Part model, mm, in its own coordinate system. Face numbers are marked on the shaded views. A direction names the side the tool comes from. Round coordinates to 2 decimals unless told otherwise and drop trailing zeros. Write each loop counter-clockwise with the first axis right and the second up, starting at its lowest first coordinate (ties: lowest second). Pieces come first, ordered by that corner, then holes. Notation, with made-up numbers: M -23.5,-21 L -2.5,-21 A18 cw -2.5,-9 Z; hole C 71.5,38 d7. An arc over 180 degrees is marked long. Answer as a JSON object with one key per item and string values. Group by question number.
1. Band-saw the part on D-D, the plane z = 9. Write the cut outline in (x, y) (3 decimals).
2. Which spindle directions (+Z, -Z, +X, -X, +Y, -Y) get a long thin tool onto all of the face, cutting with end or side? Do the marked faces 5 and 6. Say none if no direction does.
3. Two-plate mould, pull along Z, no slides. Class the marked faces 1, 2, 3 and 4: +Z half, -Z half, draft (parallel to the pull), parting line (faces both ways), or undercut.
4. Band-saw the part on C-C, the plane x = 3.25. Write the cut outline in (y, z).
5. Drill centre lines: line 1 (Z direction, x = 2.5, y = 1.25); line 2 (Y direction, x = 4.5, z = 9.25) (3 decimals); line 3 (X direction, y = 2.5, z = 1.25). Where is each one in solid material? Low to high. Write a range as from..to.
6. Band-saw the part on A-A, the plane x = 7.25. Write the cut outline in (y, z) (3 decimals).
7. Drop flat-ended pins along their axis: pin 1 (3 mm diameter, centred on y = 7, z = 3, fed in from +X); pin 2 (1.5 mm diameter, centred on x = 1.5, z = 6.5, fed in from +Y); pin 3 (1.5 mm diameter, centred on y = 4.5, z = 2.5, fed in from -X); pin 4 (1 mm diameter, centred on y = 7.5, z = 7.5, fed in from -X). Give the stop position or say it passes through.
8. Band-saw the part on B-B, the plane y = 6. Write the cut outline in (x, z), plus the area to 3 significant figures.
from build123d import *

# Parameters (mm, degrees)
BOSS_EXTRUDE2_DEPTH = 8.255
FILLET1_R           = 4.064
SKETCH2_R           = 2.07899
CUT_EXTRUDE1_DEPTH  = 11.16


with BuildPart() as part:
    # Sketch1 → Boss-Extrude2 (new body)
    with BuildSketch(Plane(origin=(0, 0, 0), x_dir=(1, 0, 0), z_dir=(0, 1, 0))):
        with BuildLine():
            Line((0, 0), (11.2268, 0))
            Line((11.2268, 0), (11.481438195, 0))
            ThreePointArc((11.481438195, 0), (11.2268, -5.08), (11.481438195, -10.16))
            Line((11.481438195, -10.16), (11.2268, -10.16))
            Line((11.2268, -10.16), (0, -10.16))
            Line((0, -10.16), (0, -8.07974))
            Line((0, -8.07974), (9.3218, -8.07974))
            Line((9.3218, -8.07974), (9.3218, -5.08))
            Line((9.3218, -5.08), (9.3218, -2.07974))
            Line((9.3218, -2.07974), (0, -2.07974))
            Line((0, -2.07974), (0, 0))
        make_face()
    extrude(amount=BOSS_EXTRUDE2_DEPTH)

    # Fillet1
    fillet1_edges = [part.edges().sort_by_distance(p)[0] for p in [
        (0, 0, 9.11987),
        (0, 0, 1.03987),
        (0, 8.255, 9.11987),
        (0, 8.255, 1.03987),
    ]]
    fillet(fillet1_edges, radius=FILLET1_R)

    # Sketch2 → Cut-Extrude1 (cut, through all)
    with BuildSketch(Plane(origin=(0, 0, 0), x_dir=(-1, 0, 0), z_dir=(0, 0, -1))):
        with Locations((-4.064, 4.191)):
            Circle(SKETCH2_R)
    extrude(amount=-CUT_EXTRUDE1_DEPTH, mode=Mode.SUBTRACT)


solid = part.part
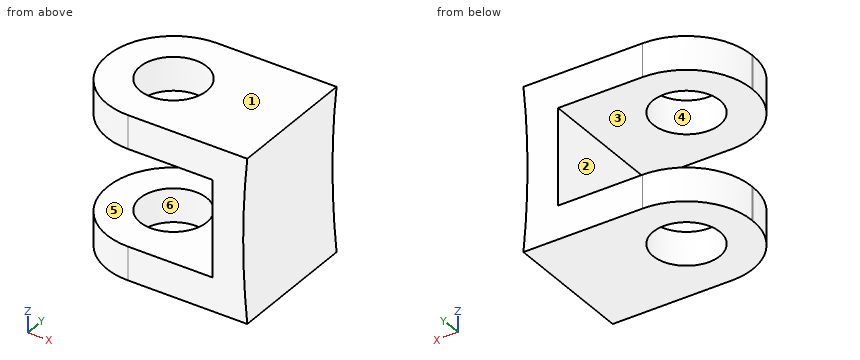
Worked answers:
{
 "1": {"outline": "M 0,4.064 A4.064 ccw 4.064,0 L 11.378,0 L 11.378,8.255 L 4.064,8.255 A4.064 ccw 0,4.191 Z; hole C 4.064,4.191 d4.158"},
 "2": {"face 5": "-X, +Y, -Y", "face 6": "+Z, -Z"},
 "3": {"face 1": "+Z half", "face 2": "undercut", "face 3": "undercut", "face 4": "draft"},
 "4": {"outline": "M 0.08,0 L 2.28,0 L 2.28,2.08 L 0.08,2.08 Z; M 0.08,8.08 L 2.28,8.08 L 2.28,10.16 L 0.08,10.16 Z; M 6.1,0 L 8.17,0 L 8.17,2.08 L 6.1,2.08 Z; M 6.1,8.08 L 8.17,8.08 L 8.17,10.16 L 6.1,10.16 Z"},
 "5": {"line 1": "z = 0..2.08, 8.08..10.16", "line 2": "y = 0..2.158, 6.224..8.255", "line 3": "x = 0.31..2.85, 5.27..11.37"},
 "6": {"outline": "M 0,0 L 8.255,0 L 8.255,2.08 L 0,2.08 Z; M 0,8.08 L 8.255,8.08 L 8.255,10.16 L 0,10.16 Z"},
 "7": {"pin 1": "stops at x = 11.35", "pin 2": "passes through", "pin 3": "stops at x = 0", "pin 4": "stops at x = 9.32"},
 "8": {"outline": "M 0.42,0 L 3.04,0 L 3.04,2.08 L 0.42,2.08 Z; M 0.42,8.08 L 3.04,8.08 L 3.04,10.16 L 0.42,10.16 Z; M 5.09,0 L 11.48,0 A50.8 cw 11.48,10.16 L 5.09,10.16 L 5.09,8.08 L 9.32,8.08 L 9.32,2.08 L 5.09,2.08 Z", "area": "48.7 mm^2"}
}
